from build123d import *

# Parameters (mm, degrees)
SKETCH_1_W          = 15
SKETCH_1_H          = 64
EXTRUDE_1_DEPTH     = 40
SKETCH_2_W          = 30.056005851
SKETCH_2_H          = 62
CUT_EXTRUDE_1_DEPTH = 39
SKETCH_3_W          = 28.51308974
SKETCH_3_H          = 3.641282023
CUT_EXTRUDE_2_DEPTH = 35
SKETCH_4_R          = 1.6
CUT_EXTRUDE_3_DEPTH = 35
SKETCH_5_W          = 1
SKETCH_5_H          = 27.039604853
EXTRUDE_2_DEPTH     = 62
SKETCH_7_W          = 23.742414222
SKETCH_7_H          = 58.772442454
CUT_EXTRUDE_5_DEPTH = 62


with BuildPart() as part:
    # 草图1 → 凸台-拉伸1 (new body)
    with BuildSketch(Plane.XY):
        with Locations((7.5, 32)):
            Rectangle(SKETCH_1_W, SKETCH_1_H)
    extrude(amount=EXTRUDE_1_DEPTH)

    # 草图2 → 切除-拉伸1 (cut)
    with BuildSketch(Plane.XY.offset(40)):
        with Locations((11.079565378, 32)):
            Rectangle(SKETCH_2_W, SKETCH_2_H)
    extrude(amount=-CUT_EXTRUDE_1_DEPTH, mode=Mode.SUBTRACT)

    # 草图3 → 切除-拉伸2 (cut)
    with BuildSketch(Plane.XY.offset(40)):
        with Locations((10.369823967, 63.629780285)):
            Rectangle(SKETCH_3_W, SKETCH_3_H)
    extrude(amount=-CUT_EXTRUDE_2_DEPTH, mode=Mode.SUBTRACT)

    # 草图4 → 切除-拉伸3 (cut)
    with BuildSketch(Plane(origin=(0, 1, 0), x_dir=(1, 0, 0), z_dir=(0, 1, 0))):
        with Locations(Location((10, -30, 0), (0, 0, 270))):
            Circle(SKETCH_4_R)
    extrude(amount=-CUT_EXTRUDE_3_DEPTH, mode=Mode.SUBTRACT)

    # 草图5 → 凸台-拉伸2 (add)
    with BuildSketch(Plane(origin=(0, 1, 0), x_dir=(1, 0, 0), z_dir=(0, 1, 0))):
        with Locations((10.105118674, -14.040486519)):
            Rectangle(SKETCH_5_W, SKETCH_5_H)
    extrude(amount=EXTRUDE_2_DEPTH)

    # 草图7 → 切除-拉伸5 (cut)
    with BuildSketch(Plane(origin=(10.605118674, 0, 0), x_dir=(0, 0, -1), z_dir=(1, 0, 0))):
        with Locations((-15.689081835, 33.613778773)):
            Rectangle(SKETCH_7_W, SKETCH_7_H)
    extrude(amount=-CUT_EXTRUDE_5_DEPTH, mode=Mode.SUBTRACT)


solid = part.part
Here's how the part is built. I have some questions about the finished solid (model axes, mm). A direction names the side the tool comes from. Give positions to 0.01 mm unless a question says otherwise; leave off trailing zeros. Order: outer loops, then holes, each group sorted by start corner. A loop starts at its lowest first (then second) coordinate and runs counter-clockwise, first axis right, second up. Notation, with made-up numbers: (-5.75, 23) -> (38.25, 23) arc R20 ccw to (38.25, 60) -> close; hole circle Ø8 at (21, -23). An arc over 180 degrees is marked (long way). Use a Markdown table: item, result. Add a question column.
Item 1: Imagine slicing it at D-D on z = 35. Please give me the cut outline in (x, y), plus the area to 3 significant figures.
Item 2: Imagine slicing it at B-B on x = 1. Please give me the cut outline in (y, z), plus the area to 3 significant figures.
Item 3: If we mould it in two halves opening along Z, with no side actions, what happens to faces 1 (the face through (5, 32, 1)), 2 (the face through (7, 1, 21)), 3 (the face through (9.03, 0.51, 28.73))? For each: pulls with the +Z half, pulls with the -Z half, needs draft (parallel to the pull), parting line crosses it, or undercut.
Item 4: Will these pins go through, and if not, where does the flat tip stop? pin 1 (5 mm diameter, centred on x = 3.5, y = 40, fed in from +Z); pin 2 (21 mm diameter, centred on y = 20, z = 12, fed in from -X); pin 3 (4.5 mm diameter, centred on x = 5.5, z = 22.5, fed in from +Y).
Item 5: Imagine slicing it at A-A on z = 30. Please give me the cut outline in (x, y).
Item 6: For faces 4 (the face through (13, 32, 1)), 5 (the face through (7, 32, 0)), 6 (the face through (0, 31.9, 0.6)), 7 (the face through (7, 63, 3)), 8 (the face through (9.605, 25, 3.5)), which set-ups out of +Z, -Z, +X, -X, +Y, -Y let a thin tool reach every point of the face, with its end or its side?
Item 7: I need wall thicknesses on line 1 (Y direction, x = 2.5, z = 28.5); line 2 (X direction, y = 0.65, z = 30). Which ranges of each line are inside material? Lowest first, please.
Item 8: Imagine slicing it at C-C on y = 45.5. Please give me the cut outline in (x, z), plus the area to 3 significant figures.
Data:
| question | item | result |
|---|---|---|
| 1 | outline | (0, 0) -> (15, 0) -> (15, 1) -> (0, 1) -> close |
| 1 | area | 15.0 mm² |
| 2 | outline | (0, 0) -> (64, 0) -> (64, 5) -> (63, 5) -> (63, 1) -> (1, 1) -> (1, 40) -> (0, 40) -> close |
| 2 | area | 107 mm² |
| 3 | face 1 | pulls with the +Z half |
| 3 | face 2 | needs draft |
| 3 | face 3 | undercut |
| 4 | pin 1 | stops at z = 1 |
| 4 | pin 2 | stops at x = 9.61 |
| 4 | pin 3 | stops at y = 1 |
| 5 | outline | (0, 0) -> (8.4, 0) -> (8.4, 1) -> (0, 1) -> close; (11.6, 0) -> (15, 0) -> (15, 1) -> (11.6, 1) -> close |
| 6 | face 4 | +Z, +X |
| 6 | face 5 | -Z, +X, -X, +Y, -Y |
| 6 | face 6 | +Z, -Z, -X, +Y, -Y |
| 6 | face 7 | +Z |
| 6 | face 8 | +Z, -X |
| 7 | line 1 | y = 0 to 1 |
| 7 | line 2 | x = 0 to 8.4, 11.6 to 15 |
| 8 | outline | (0, 0) -> (15, 0) -> (15, 1) -> (10.61, 1) -> (10.61, 3.82) -> (9.61, 3.82) -> (9.61, 1) -> (0, 1) -> close |
| 8 | area | 17.8 mm² |
